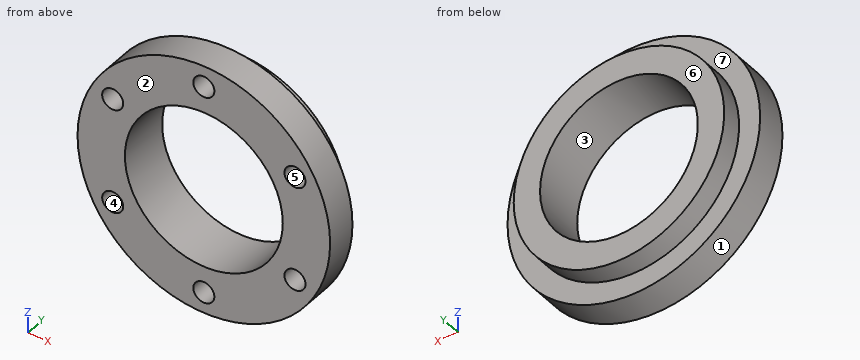
```python
from build123d import *

# Parameters (mm, degrees)
SKETCH1_R           = 12
SKETCH1_R_2         = 7.5
BOSS_EXTRUDE1_DEPTH = 3
SKETCH2_R           = 1
CUT_EXTRUDE1_DEPTH  = 2.2
SKETCH3_R           = 10
SKETCH3_R_2         = 7.5
BOSS_EXTRUDE2_DEPTH = 2


with BuildPart() as part:
    # Sketch1 → Boss-Extrude1 (new body)
    with BuildSketch(Plane(origin=(0, 0, 0), x_dir=(1, 0, 0), z_dir=(0, 1, 0))):
        Circle(SKETCH1_R)
        Circle(SKETCH1_R_2, mode=Mode.SUBTRACT)
    extrude(amount=BOSS_EXTRUDE1_DEPTH)

    # Sketch2 → Cut-Extrude1 (cut)
    with BuildSketch(Plane.XZ):
        with Locations((0, 10)):
            Circle(SKETCH2_R)
        with Locations((-8.660254038, 5)):
            Circle(SKETCH2_R)
        with Locations((-8.660254038, -5)):
            Circle(SKETCH2_R)
        with Locations((0, -10)):
            Circle(SKETCH2_R)
        with Locations((8.660254038, -5)):
            Circle(SKETCH2_R)
        with Locations((8.660254038, 5)):
            Circle(SKETCH2_R)
    extrude(amount=-CUT_EXTRUDE1_DEPTH, mode=Mode.SUBTRACT)

    # Sketch3 → Boss-Extrude2 (add)
    with BuildSketch(Plane(origin=(0, 3, 0), x_dir=(1, 0, 0), z_dir=(0, 1, 0))):
        Circle(SKETCH3_R)
        Circle(SKETCH3_R_2, mode=Mode.SUBTRACT)
    extrude(amount=BOSS_EXTRUDE2_DEPTH)


solid = part.part
```
Input: part model. Units: mm. Frame: model coordinates. Face numbers are marked on the shaded views. A direction names the side the tool comes from. Give positions to 0.01 mm unless a question says otherwise; leave off trailing zeros. Order: outer loops, then holes, each group sorted by start corner. A loop starts at its lowest first (then second) coordinate and runs counter-clockwise, first axis right, second up. Notation, with made-up numbers: (-13.5, -28.5) -> (40.5, -28.5) arc R10 cw to (40.5, -15.5) -> close; hole circle Ø7 at (73, 47). An arc over 180 degrees is marked (long way). Write each question's results on one line, items separated by ' | '. Start each with the question number.
Item 1: Line query: line 1 (Z direction, x = 0, y = 0.55); line 2 (X direction, y = 1.4, z = 0); line 3 (X direction, y = 2.05, z = -4.25). Output: solid intervals per line, ascending.
Item 2: Cut plane A-A on y = 1.55. Return the cut outline in (x, z).
Item 3: Cut plane B-B on x = 0. Return the cut outline in (y, z).
Item 4: Set-up query: the marked faces 5, 6 and 7. Return all of +Z, -Z, +X, -X, +Y, -Y with unobstructed straight access to the full face (end or side cutting, diameter ignored); none if empty.
Item 5: Cut plane C-C on z = -3. Return the cut outline in (x, y).
Item 6: Cut plane D-D on x = 8. Return the cut outline in (y, z), then the cut area to 3 significant figures.
Item 7: Contact query for flat-ended pins moving along their axis: P1, Ø1.8, axis at x = 8.66, z = 5, coming from the -Y side; P2, Ø2, axis at y = 3.5, z = -3.5, coming from the +X side. Output: stop coordinate, or through.
Item 8: Mould query, pull axis Z, two halves, no side actions, for the marked faces 1, 2, 3 and 4. Classes: pulls with the +Z half, pulls with the -Z half, needs draft (parallel to the pull), parting line crosses it, or undercut.
Established:
1) line 1: -12 to -11, -9 to -7.5, 7.5 to 9, 11 to 12 | line 2: -12 to -7.5, 7.5 to 12 | line 3: -11.22 to -9.32, -8 to -6.18, 6.18 to 8, 9.32 to 11.22
2) outline: circle Ø24 at (0, 0); hole circle Ø2 at (-8.66, -5); hole circle Ø2 at (-8.66, 5); hole circle Ø15 at (0, 0); hole circle Ø2 at (0, -10); hole circle Ø2 at (0, 10); hole circle Ø2 at (8.66, -5); hole circle Ø2 at (8.66, 5)
3) outline: (0, -12) -> (3, -12) -> (3, -10) -> (5, -10) -> (5, -7.5) -> (0, -7.5) -> (0, -9) -> (2.2, -9) -> (2.2, -11) -> (0, -11) -> close; (0, 7.5) -> (5, 7.5) -> (5, 10) -> (3, 10) -> (3, 12) -> (0, 12) -> (0, 11) -> (2.2, 11) -> (2.2, 9) -> (0, 9) -> close
4) face 5: -Y | face 6: +Z, -Z, +X, -X, +Y | face 7: +Y
5) outline: (-11.62, 0) -> (-6.87, 0) -> (-6.87, 5) -> (-9.54, 5) -> (-9.54, 3) -> (-11.62, 3) -> close; (6.87, 0) -> (11.62, 0) -> (11.62, 3) -> (9.54, 3) -> (9.54, 5) -> (6.87, 5) -> close
6) outline: (0, -8.94) -> (3, -8.94) -> (3, -6) -> (5, -6) -> (5, 6) -> (3, 6) -> (3, 8.94) -> (0, 8.94) -> (0, 5.75) -> (2.2, 5.75) -> (2.2, 4.25) -> (0, 4.25) -> (0, -4.25) -> (2.2, -4.25) -> (2.2, -5.75) -> (0, -5.75) -> close | area: 71.1 mm^2
7) P1: y = 2.2 | P2: x = 11.71
8) face 1: parting line crosses it | face 2: needs draft | face 3: undercut | face 4: undercut
